Autodesk Inventor part; units mm, degrees
ref_plane "YZ Plane" through (0, 0, 0) normal (1, 0, 0) x (0, 1, 0)
ref_plane "XZ Plane" through (0, 0, 0) normal (0, 1, 0) x (-1, 0, 0)
ref_plane "XY Plane" through (0, 0, 0) normal (0, 0, 1) x (1, 0, 0)
sketch "Sketch2" plane through (0, 0, 0) normal (0, 0, 1) x (1, 0, 0)
  line L0 (-75, -25) -> (75, -25)
  line L1 (75, -25) -> (75, 25)
  line L2 (75, 25) -> (-75, 25)
  line L3 (-75, 25) -> (-75, -25)
  line L4 (-75, -25) -> (75, 25) construction
  line L5 (75, -25) -> (-75, 25) construction
  point P0 (0, 0)
  dimension "d1" = 150
  dimension "d2" = 50
extrude "Extrusion1" add sketch "Sketch2" along normal mid plane 10
sketch "Sketch3" plane through (0, 0, 5) normal (0, 0, 1) x (1, 0, 0)
  line L0 (-75, 25) -> (-75, -25)
  line L1 (75, 25) -> (-75, 25)
  point P0 (0, 0)
  point P1 (-65, 0)
  dimension "d40" = 10
  dimension "d43" = 25
hole "Hole1" at (-65, 0, 5) direction (0, 0, -1) diameter 6.6 depth 14.2 tip angle 118
sketch "Sketch4" plane through (0, 0, 5) normal (0, 0, 1) x (1, 0, 0)
  line L0 (-75, 25) -> (-75, -25)
  line L1 (75, 25) -> (-75, 25)
  point P0 (0, 0)
  point P1 (-45, 5)
  dimension "d41" = 30
  dimension "d42" = 20
hole "Hole2" at (-45, 5, 5) direction (0, 0, -1) diameter 9 depth 14.2 tip angle 118
sketch "Sketch5" plane through (0, 0, 5) normal (0, 0, 1) x (1, 0, 0)
  line L0 (-75, 25) -> (-75, -25)
  line L1 (75, 25) -> (-75, 25)
  point P0 (0, 0)
  point P1 (-25, 5)
  dimension "d44" = 50
  dimension "d45" = 20
hole "Hole3" at (-25, 5, 5) direction (0, 0, -1) diameter 6.6 depth 14.2 tip angle 118
sketch "Sketch6" plane through (0, 0, 5) normal (0, 0, 1) x (1, 0, 0)
  line L0 (-75, 25) -> (-75, -25)
  line L1 (75, 25) -> (-75, 25)
  point P0 (0, 0)
  point P1 (5, 5)
  dimension "d46" = 80
  dimension "d47" = 20
hole "Hole4" at (5, 5, 5) direction (0, 0, -1) diameter 8 depth 14.2 tip angle 118
sketch "Sketch7" plane through (0, 0, 5) normal (0, 0, 1) x (1, 0, 0)
  line L0 (-75, 25) -> (-75, -25)
  line L1 (75, 25) -> (-75, 25)
  point P0 (0, 0)
  point P1 (25, 5)
  dimension "d48" = 100
  dimension "d49" = 20
hole "Hole5" at (25, 5, 5) direction (0, 0, -1) diameter 12 depth 14.2 tip angle 118
properties part number "홀간 거리 확인 파트-7" material "SS400"
Design review of the part built by this model. Coordinates are the model's own, in mm. Round coordinates to 2 decimals unless told otherwise and drop trailing zeros. Order: outer loops, then holes, each group sorted by start corner. A loop starts at its lowest first (then second) coordinate and runs counter-clockwise, first axis right, second up.
1) Draft analysis for pull direction Y (two halves, no side actions). For faces 1 (the flat face through (-75, 0, 0)), 2 (the flat face through (-1, -25, 0)), 3 (the cylindrical face through (28.65, 9.76, -0.07)), 4 (the cylindrical face through (-68.27, 0.43, -0.07)), state which applies: released by +Y, released by -Y, zero draft, split by the parting line, or undercut.
The answers:
face 1: zero draft
face 2: released by -Y
face 3: undercut
face 4: undercut
2) Consider section D-D (x = 5). State the section outline as (y, z) points, plus the area to 3 significant figures.
The answers:
outline: (-25, -5) - (1, -5) - (1, 5) - (-25, 5) - close; (9, -5) - (25, -5) - (25, 5) - (9, 5) - close
area: 420 mm2
3) For L1, parallel to X at y = 5, z = -0.25; L2, parallel to Y at x = 25, z = -0.75; L3, parallel to X at y = 0, z = 0.5, list the stretches that pass through material, from the lowest coordinate up.
The answers:
L1: x = -75 to -49.5, -40.5 to -28.3, -21.7 to 1, 9 to 19, 31 to 75
L2: y = -25 to -1, 11 to 25
L3: x = -75 to -68.3, -61.7 to 21.68, 28.32 to 75
4) Consider section A-A (z = -0.75). State the section outline as (x, y) points.
The answers:
outline: (-75, -25) - (75, -25) - (75, 25) - (-75, 25) - close; hole circle Ø6.6 at (-65, 0); hole circle Ø9 at (-45, 5); hole circle Ø6.6 at (-25, 5); hole circle Ø8 at (5, 5); hole circle Ø12 at (25, 5)
5) Clearance check with a flat-ended pin moving along its axis: pin 1 Ø4 at (x, y) = (-65, 0) entering from -Z. State where the tip first meets the part, or that it passes through.
The answers:
pin 1: passes through
6) Consider section C-C (y = 5). State the section outline as (x, z) points.
The answers:
outline: (-75, -5) - (-49.5, -5) - (-49.5, 5) - (-75, 5) - close; (-40.5, -5) - (-28.3, -5) - (-28.3, 5) - (-40.5, 5) - close; (-21.7, -5) - (1, -5) - (1, 5) - (-21.7, 5) - close; (9, -5) - (19, -5) - (19, 5) - (9, 5) - close; (31, -5) - (75, -5) - (75, 5) - (31, 5) - close
7) Consider section B-B (x = 25). State the section outline as (y, z) points, plus the area to 3 significant figures.
The answers:
outline: (-25, -5) - (-1, -5) - (-1, 5) - (-25, 5) - close; (11, -5) - (25, -5) - (25, 5) - (11, 5) - close
area: 380 mm2
